Read the model definition and answer for the solid it produces. Units are mm, in the model's axes. A direction names the side the tool comes from. Coordinates: 2 decimals unless noted, no trailing zeros. Order: outer loops, then holes, each group sorted by start corner. A loop starts at its lowest first (then second) coordinate and runs counter-clockwise, first axis right, second up.
```python
from build123d import *

# Parameters (mm, degrees)
SKETCH1_W           = 28.96
SKETCH1_H           = 11
BOSS_EXTRUDE1_DEPTH = 7.5
SKETCH2_W           = 8.255
SKETCH2_H           = 7.5
BOSS_EXTRUDE2_DEPTH = 23.8
SKETCH3_W           = 28.96
SKETCH3_H           = 7.5
BOSS_EXTRUDE3_DEPTH = 8
SKETCH4_W           = 4.56
SKETCH4_H           = 7.5
CUT_EXTRUDE1_DEPTH  = 5
SKETCH5_R           = 1.92
CUT_EXTRUDE2_DEPTH  = 10


with BuildPart() as part:
    # Sketch1 → Boss-Extrude1 (new body)
    with BuildSketch(Plane.XY):
        with Locations((-4.078230088, 25.589734513)):
            Rectangle(SKETCH1_W, SKETCH1_H)
    extrude(amount=BOSS_EXTRUDE1_DEPTH)

    # Sketch2 → Boss-Extrude2 (add)
    with BuildSketch(Plane(origin=(0, 31.089734513, 0), x_dir=(1, 0, 0), z_dir=(0, 1, 0))):
        with Locations((-14.430730088, -3.75)):
            Rectangle(SKETCH2_W, SKETCH2_H)
        with Locations((6.274269912, -3.75)):
            Rectangle(SKETCH2_W, SKETCH2_H)
    extrude(amount=BOSS_EXTRUDE2_DEPTH)

    # Sketch3 → Boss-Extrude3 (add)
    with BuildSketch(Plane(origin=(0, 54.889734513, 0), x_dir=(1, 0, 0), z_dir=(0, 1, 0))):
        with Locations((-4.078230088, -3.75)):
            Rectangle(SKETCH3_W, SKETCH3_H)
    extrude(amount=BOSS_EXTRUDE3_DEPTH)

    # Sketch4 → Cut-Extrude1 (cut)
    with BuildSketch(Plane(origin=(0, 31.089734513, 0), x_dir=(1, 0, 0), z_dir=(0, 1, 0))):
        with Locations((-4.078230088, -3.75)):
            Rectangle(SKETCH4_W, SKETCH4_H)
    extrude(amount=-CUT_EXTRUDE1_DEPTH, mode=Mode.SUBTRACT)

    # Sketch5 → Cut-Extrude2 (cut)
    with BuildSketch(Plane.XY.offset(7.5)):
        with Locations((-14.703230088, 43.409734513)):
            Circle(SKETCH5_R)
        with Locations((6.546769912, 43.409734513)):
            Circle(SKETCH5_R)
    extrude(amount=-CUT_EXTRUDE2_DEPTH, mode=Mode.SUBTRACT)


solid = part.part
```
1) Straight lines are drawn through the part: line 1 (X direction, y = 43.5, z = 0.75); line 2 (Y direction, x = -6.5, z = 4.5); line 3 (Y direction, x = -2, z = 6.25). For each, find the intervals that lie inside material, in ascending order.
A:
line 1: x = -18.56 to -16.62, -12.79 to -10.3, 2.15 to 4.63, 8.46 to 10.4
line 2: y = 20.09 to 31.09, 54.89 to 62.89
line 3: y = 20.09 to 26.09, 54.89 to 62.89
2) A cutting plane is placed at C-C, the plane z = 2.5. Determine the outline of the cut face in (x, y).
A:
outline: (-18.56, 20.09) - (10.4, 20.09) - (10.4, 62.89) - (-18.56, 62.89) - close; hole circle Ø3.84 at (-14.7, 43.41); hole (-10.3, 31.09) - (-6.36, 31.09) - (-6.36, 26.09) - (-1.8, 26.09) - (-1.8, 31.09) - (2.15, 31.09) - (2.15, 54.89) - (-10.3, 54.89) - close; hole circle Ø3.84 at (6.55, 43.41)
3) Which of the six approach directions +Z, -Z, +X, -X, +Y, -Y give full straight-line access (tool end or side, diameter ignored) to faces 5 (the flat face through (-11, 41, 0)), 6 (the flat face through (-10.303, 43, 4))?
A:
face 5: -Z, +X, -X, +Y, -Y
face 6: +Z, -Z
4) A cutting plane is placed at A-A, the plane x = -3.25. Determine the outline of the cut face in (y, z), and give its area (3 significant figures).
A:
outline: (20.09, 0) - (26.09, 0) - (26.09, 7.5) - (20.09, 7.5) - close; (54.89, 0) - (62.89, 0) - (62.89, 7.5) - (54.89, 7.5) - close
area: 105 mm2
5) A cutting plane is placed at B-B, the plane y = 50. Determine the outline of the cut face in (x, z).
A:
outline: (-18.56, 0) - (-10.3, 0) - (-10.3, 7.5) - (-18.56, 7.5) - close; (2.15, 0) - (10.4, 0) - (10.4, 7.5) - (2.15, 7.5) - close
6) A flat-ended cylindrical pin translates along its axis: pin 1 Ø5 at (x, y) = (-2, 47.5) entering from +Z. Find the tip coordinate at first contact, or state that the pin passes through.
A:
pin 1: passes through
7) Determine the mould class of faces 1 (the flat face through (2.147, 43, 4)), 2 (the cylindrical face through (-12.872, 43.986, 3.802)), 3 (the flat face through (-4, 20.09, 4)), 4 (the flat face through (10.402, 41, 4)) for opening direction Y: pulls with the +Y half, pulls with the -Y half, needs draft (parallel to the pull), parting line crosses it, or undercut.
A:
face 1: undercut
face 2: undercut
face 3: pulls with the -Y half
face 4: needs draft
